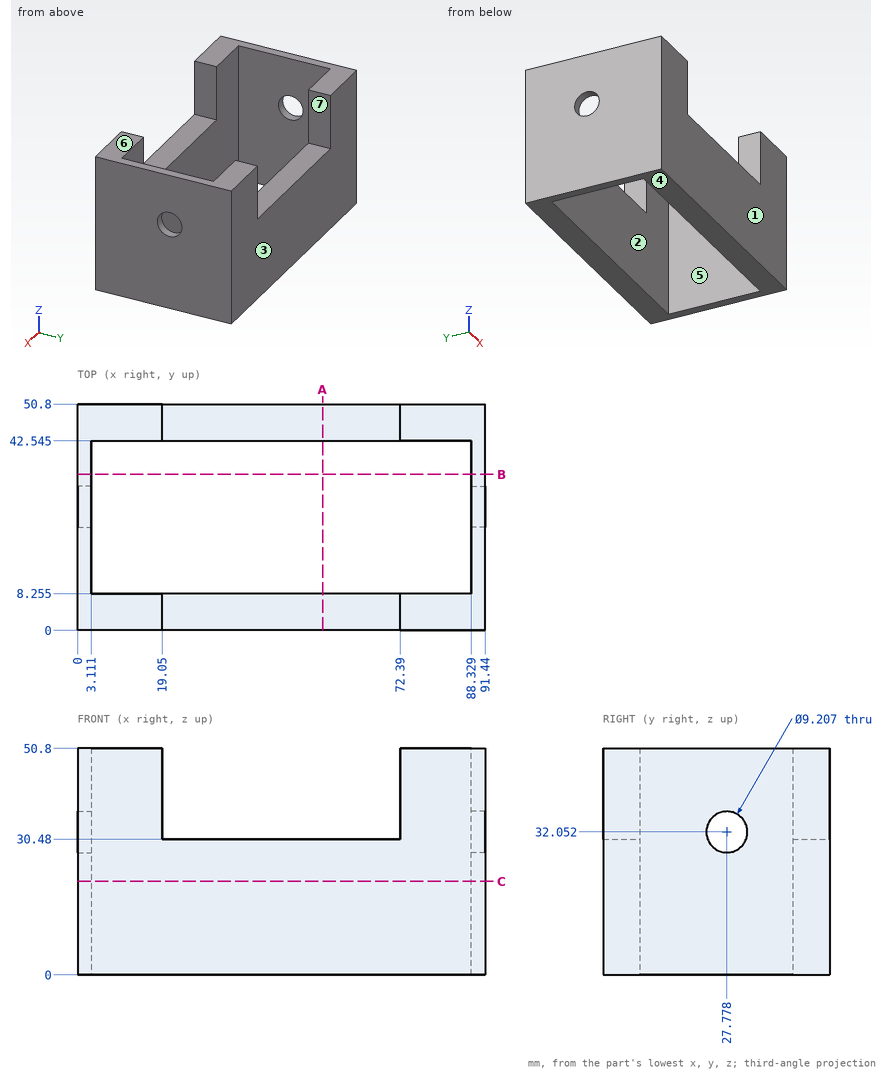
Part print with two shaded views. Sizes in mm from the minimum x, y, z corner. A direction names the side the tool comes from. Round coordinates to 2 decimals unless told otherwise and drop trailing zeros. Order: outer loops, then holes, each group sorted by start corner. A loop starts at its lowest first (then second) coordinate and runs counter-clockwise, first axis right, second up.
(1) Band-saw the part on A-A (x = 55). List the corners of the cut face in (y, z) (1 decimal), then the cut area to 3 significant figures.
(2) Band-saw the part on C-C (z = 21). List the corners of the cut face in (x, y) (1 decimal).
(3) Band-saw the part on B-B (y = 35). List the corners of the cut face in (x, z), then the cut area to 3 significant figures.
(4) Pin check, flat tips, straight feed: pin 1 (9 mm diameter, centred on x = 40, y = 45.5, fed in from +Z); pin 2 (7.5 mm diameter, centred on y = 27.78, z = 32.05, fed in from -X). Stop position of each tip, or through.
(5) Pull direction Y, two halves, no side cores. Call the marked faces 1, 2, 3 and 4: released by +Y, released by -Y, zero draft, split by the parting line, or undercut.
(6) 3-axis set-ups, long thin cutter, end or side, ignore diameter. For the marked faces 5, 6 and 7: which of +Z, -Z, +X, -X, +Y, -Y reach the whole face in a straight line?
(7) Drill centre lines: line 1 (X direction, y = 21, z = 8); line 2 (Y direction, x = 52.5, z = 11) (1 decimal); line 3 (Z direction, x = 59, y = 48). Where is each one in solid material? Low to high.
Verdict:
1. outline: (0, 0) - (8.3, 0) - (8.3, 30.5) - (0, 30.5) - close; (42.5, 0) - (50.8, 0) - (50.8, 30.5) - (42.5, 30.5) - close
1. area: 503 mm2
2. outline: (0, 0) - (91.4, 0) - (91.4, 50.8) - (0, 50.8) - close; hole (3.1, 8.3) - (88.3, 8.3) - (88.3, 42.5) - (3.1, 42.5) - close
3. outline: (0, 0) - (3.11, 0) - (3.11, 50.8) - (0, 50.8) - close; (88.33, 0) - (91.44, 0) - (91.44, 50.8) - (88.33, 50.8) - close
3. area: 316 mm2
4. pin 1: stops at z = 30.48
4. pin 2: passes through
5. face 1: released by -Y
5. face 2: undercut
5. face 3: released by +Y
5. face 4: zero draft
6. face 5: +Z, -Z
6. face 6: +Z, +X, -X, +Y, -Y
6. face 7: +Z, +Y, -Y
7. line 1: x = 0 to 3.11, 88.33 to 91.44
7. line 2: y = 0 to 8.3, 42.5 to 50.8
7. line 3: z = 0 to 30.48
